from build123d import *
from OCP.BRepFilletAPI import BRepFilletAPI_MakeChamfer

# Parameters (mm, degrees)
SKETCH1_W           = 2.54
SKETCH1_H           = 2.54
BOSS_EXTRUDE1_DEPTH = 2.54
SKETCH2_W           = 0.65
SKETCH2_H           = 0.65
BOSS_EXTRUDE2_DEPTH = 5.7
SKETCH3_W           = 0.65
SKETCH3_H           = 0.65
BOSS_EXTRUDE3_DEPTH = 3.1
CHAMFER1_SIZE       = 0.091719204
CHAMFER1_SIZE2      = 0.3
CHAMFER2_SIZE       = 0.3
CHAMFER2_SIZE2      = 0.091719204
CHAMFER3_SIZE       = 0.7
CHAMFER3_SIZE2      = 0.341412812


with BuildPart() as part:
    # Sketch1 → Boss-Extrude1 (new body)
    with BuildSketch(Plane(origin=(1.27, 0, 0), x_dir=(0, 0, -1), z_dir=(1, 0, 0))):
        with Locations((0, 1.27)):
            Rectangle(SKETCH1_W, SKETCH1_H)
    extrude(amount=-BOSS_EXTRUDE1_DEPTH)

    # Sketch2 → Boss-Extrude2 (add)
    with BuildSketch(Plane(origin=(0, 2.54, 0), x_dir=(-1, 0, 0), z_dir=(0, 1, 0))):
        Rectangle(SKETCH2_W, SKETCH2_H)
    extrude(amount=BOSS_EXTRUDE2_DEPTH)

    # Sketch3 → Boss-Extrude3 (add)
    with BuildSketch(Plane.XZ):
        Rectangle(SKETCH3_W, SKETCH3_H)
    extrude(amount=BOSS_EXTRUDE3_DEPTH)

    # Chamfer1
    chamfer1_edges = [part.edges().sort_by_distance(p)[0] for p in [
        (0.325, 8.24, 0),
        (0, 8.24, -0.325),
        (-0.325, 8.24, 0),
        (0, 8.24, 0.325),
    ]]
    chamfer1_side = [part.faces().sort_by_distance(p)[0] for p in [
        (0, 8.24, 0),
    ]]
    chamfer(chamfer1_edges, length=CHAMFER1_SIZE, length2=CHAMFER1_SIZE2, reference=chamfer1_side[0])

    # Chamfer2
    chamfer2_edges = [part.edges().sort_by_distance(p)[0] for p in [
        (0, -3.1, -0.325),
        (0.325, -3.1, 0),
        (0, -3.1, 0.325),
        (-0.325, -3.1, 0),
    ]]
    chamfer2_side = [part.faces().sort_by_distance(p)[0] for p in [
        (0, -3.1, 0),
    ]]
    chamfer(chamfer2_edges, length=CHAMFER2_SIZE, length2=CHAMFER2_SIZE2, reference=chamfer2_side[0])

    # Chamfer3: one chamfer whose edges measure the first distance from different faces: ONE call of the kernel's chamfer builder (chamfer() names one face for all edges)
    chamfer3_edges_1 = [part.edges().sort_by_distance(p)[0] for p in [
        (-1.27, 1.27, -1.27),
        (-1.27, 2.54, 0),
        (-1.27, 1.27, 1.27),
    ]]
    chamfer3_side_1 = [part.faces().sort_by_distance(p)[0] for p in [
        (-1.27, 1.27, 0),
    ]]
    chamfer3_edges_2 = [part.edges().sort_by_distance(p)[0] for p in [
        (1.27, 2.54, 0),
    ]]
    chamfer3_side_2 = [part.faces().sort_by_distance(p)[0] for p in [
        (0, 2.54, -1.234078976),
    ]]
    chamfer3_edges_3 = [part.edges().sort_by_distance(p)[0] for p in [
        (1.27, 1.27, -1.27),
    ]]
    chamfer3_side_3 = [part.faces().sort_by_distance(p)[0] for p in [
        (0, 1.27, -1.27),
    ]]
    chamfer3_edges_4 = [part.edges().sort_by_distance(p)[0] for p in [
        (1.27, 1.27, 1.27),
    ]]
    chamfer3_side_4 = [part.faces().sort_by_distance(p)[0] for p in [
        (0, 1.27, 1.27),
    ]]
    chamfer3 = BRepFilletAPI_MakeChamfer(part.part.solid().wrapped)
    for e in chamfer3_edges_1:
        chamfer3.Add(CHAMFER3_SIZE, CHAMFER3_SIZE2, e.wrapped, chamfer3_side_1[0].wrapped)  # the first distance lies on this face
    for e in chamfer3_edges_2:
        chamfer3.Add(CHAMFER3_SIZE, CHAMFER3_SIZE2, e.wrapped, chamfer3_side_2[0].wrapped)  # the first distance lies on this face
    for e in chamfer3_edges_3:
        chamfer3.Add(CHAMFER3_SIZE, CHAMFER3_SIZE2, e.wrapped, chamfer3_side_3[0].wrapped)  # the first distance lies on this face
    for e in chamfer3_edges_4:
        chamfer3.Add(CHAMFER3_SIZE, CHAMFER3_SIZE2, e.wrapped, chamfer3_side_4[0].wrapped)  # the first distance lies on this face
    add(Compound.cast(chamfer3.Shape()), mode=Mode.REPLACE)


solid = part.part
Read the model definition and answer for the solid it produces. Units are mm, in the model's axes. Coordinates: 2 decimals unless noted, no trailing zeros. Write each loop counter-clockwise with the first axis right and the second up, starting at its lowest first coordinate (ties: lowest second). Pieces come first, ordered by that corner, then holes. Notation, with made-up numbers: (81, -4) - (132, -4) arc R17 ccw to (132, 1) - close; hole circle Ø1 at (44, -5.75). An arc over 180 degrees is marked (long way). One line per question, with ' | ' between items.
Q1. Find section B-B, the plane y = 5.5. Write down the section's boundary in (x, z) (3 decimals), plus the area to 4 significant figures.
Result set:
outline: (-0.325, -0.325) - (0.325, -0.325) - (0.325, 0.325) - (-0.325, 0.325) - close | area: 0.4225 mm^2
Q2. Consider L1, parallel to X at y = -0.5, z = -0.25 (3 decimals); L2, parallel to Y at x = -0.4, z = -0.25. Determine where each line is inside the solid, lowest interval first. Write a range as [from, to].
Result set:
L1: [-0.325, 0.325] | L2: [0, 2.54]
Q3. Each of these flat-tipped pins is pushed along its axis until it touches: P1, Ø0.7, axis at y = -1, z = 0, coming from the -X side (3 decimals); P2, Ø1.3, axis at x = 0.5, z = 0.5, coming from the -Y side; P3, Ø0.7, axis at x = 0, y = -2, coming from the -Z side (3 decimals). Where does it stop, or does it pass through?
Result set:
P1: x = -0.325 | P2: y = -3.1 | P3: z = -0.325
Q4. Find section A-A, the plane z = -0.45. Write down the section's boundary in (x, y).
Result set:
outline: (-1.27, 0) - (1.27, 0) - (1.27, 2.2) - (0.57, 2.54) - (-0.93, 2.54) - (-1.27, 1.84) - close
